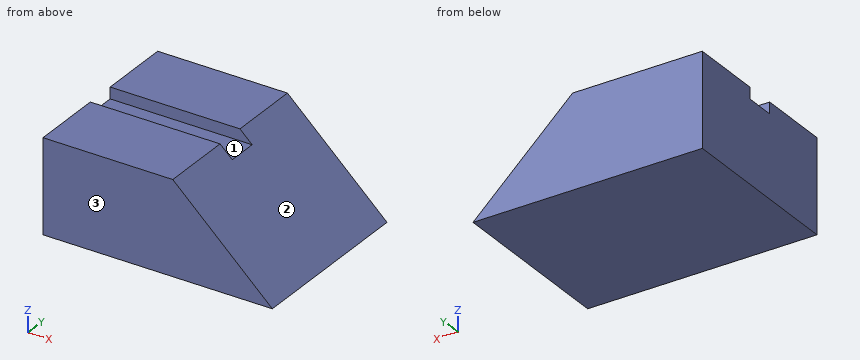
from build123d import *

# Parameters (mm, degrees)
F0_W     = 137.114138
F0_H     = 104.813702
F1_DEPTH = 55.88
F3_DEPTH = 104.814702
F4_W     = 18.162367
F4_H     = 6.841612
F5_DEPTH = 137.115137


with BuildPart() as f1:
    # F0 (on Top) → F1 (new body)
    with BuildSketch(Plane.XY):
        Rectangle(F0_W, F0_H)
    extrude(amount=F1_DEPTH)

    # F2 (on face) → F3 (cut, through all)
    with BuildSketch(Plane.XZ.offset(52.406851)):
        Polygon((68.557069, 0), (68.557069, 55.88), (9.029833, 55.88), align=None)
    extrude(amount=-F3_DEPTH, mode=Mode.SUBTRACT)

    # F4 (on face) → F5 (cut, through all)
    with BuildSketch(Plane(origin=(-68.557069, 0, 0), x_dir=(0, -1, 0), z_dir=(-1, 0, 0))):
        with Locations((0.095591, 52.459194)):
            Rectangle(F4_W, F4_H)
    extrude(amount=-F5_DEPTH, mode=Mode.SUBTRACT)


solid = f1.part
Work out the finished part from the listing and answer in its coordinate system (mm). Face numbers are marked on the shaded views. Coordinates: 2 decimals unless noted, no trailing zeros. Loops run counter-clockwise (first coordinate to the right, second up) from the corner with the lowest first, then second, coordinate; pieces in that order, holes last. Notation, with made-up numbers: (54, -32.75) -> (74, -32.75) arc R11 cw to (74, -20.75) -> close; hole circle Ø7 at (-3, 71.5). An arc over 180 degrees is marked (long way). Write each question's results on one line, items separated by ' | '. Start each with the question number.
1) The mould has two halves that part along Y. Classify the marked faces 1, 2 and 3: pulls with the +Y half, pulls with the -Y half, needs draft (parallel to the pull), parting line crosses it, or undercut.
2) Find section B-B on z = 52.5. Determine the outline of the cut face in (x, y).
3) Find section A-A on x = -47.5. Determine the outline of the cut face in (y, z), then the cut area to 3 significant figures.
4) Find section C-C on y = 3.5. Determine the outline of the cut face in (x, z), then the cut area to 3 significant figures.
5) Consider line 1 along Y through (x, z) = (-26, 49.5); line 2 along Z through (x, y) = (61, 23); line 3 along X through (y, z) = (-33.5, 17.5). Determine where each line is inside the solid, lowest interval first.
6) Flat-ended cylindrical pins translate along their axes: P1, Ø3, axis at y = 37.5, z = 50, coming from the +X side; P2, Ø14.5, axis at x = -22.5, y = 1.5, coming from the +Z side; P3, Ø8, axis at x = 1.5, y = -40.5, coming from the -Z side; P4, Ø4, axis at y = -37, z = 20, coming from the +X side. Find the tip coordinate at first contact, or state that the pin passes through.
7) Find section D-D on z = 46. Determine the outline of the cut face in (x, y).
Response values:
1) face 1: undercut | face 2: needs draft | face 3: pulls with the -Y half
2) outline: (-68.56, -52.41) -> (12.63, -52.41) -> (12.63, -9.18) -> (-68.56, -9.18) -> close; (-68.56, 8.99) -> (12.63, 8.99) -> (12.63, 52.41) -> (-68.56, 52.41) -> close
3) outline: (-52.41, 0) -> (52.41, 0) -> (52.41, 55.88) -> (8.99, 55.88) -> (8.99, 49.04) -> (-9.18, 49.04) -> (-9.18, 55.88) -> (-52.41, 55.88) -> close | area: 5,730 mm^2
4) outline: (-68.56, 0) -> (68.56, 0) -> (16.32, 49.04) -> (-68.56, 49.04) -> close | area: 5,440 mm^2
5) line 1: y = -52.41 to -9.18, 8.99 to 52.41 | line 2: z = 0 to 7.09 | line 3: x = -68.56 to 49.91
6) P1: stops at x = 16.89 | P2: stops at z = 49.04 | P3: stops at z = 0 | P4: stops at x = 49.38
7) outline: (-68.56, -52.41) -> (19.55, -52.41) -> (19.55, 52.41) -> (-68.56, 52.41) -> close
